Geometry: final body of the model. Coordinates: model frame, mm. A direction names the side the tool comes from. Give positions to 0.01 mm unless a question says otherwise; leave off trailing zeros. Order: outer loops, then holes, each group sorted by start corner. A loop starts at its lowest first (then second) coordinate and runs counter-clockwise, first axis right, second up. Notation, with made-up numbers: (-6.5, 8) - (39.5, 8) arc R28 cw to (39.5, 31) - close; hole circle Ø6 at (23, 81.5). An arc over 180 degrees is marked (long way). Use one line per item in the form item = value.
from build123d import *

# Parameters (mm, degrees)
BOSS_EXTRUDE1_DEPTH = 12.3
SKETCH2_W           = 2.17
SKETCH2_H           = 2.05
CUT_EXTRUDE1_DEPTH  = 4
FILLET1_R           = 2.15
SKETCH4_W           = 3
SKETCH4_H           = 1
BOSS_EXTRUDE2_DEPTH = 1
BOSS_EXTRUDE3_DEPTH = 3
CUT_EXTRUDE2_DEPTH  = 14.994303425


with BuildPart() as part:
    # Sketch1 → Boss-Extrude1 (new body)
    with BuildSketch(Plane(origin=(0, 0, 0), x_dir=(0, 0, -1), z_dir=(1, 0, 0))):
        with BuildLine():
            Line((0, 0.2), (0, 0.4))
            Line((0, 0.4), (0.303108891, 0.575))
            Line((0.303108891, 0.575), (0.303108891, 5.8))
            Line((0.303108891, 5.8), (3.303108891, 5.8))
            Line((3.303108891, 5.8), (3.303108891, 0))
            Line((3.303108891, 0), (0.2, 0))
            ThreePointArc((0.2, 0), (0.058578644, 0.058578644), (0, 0.2))
        make_face()
    extrude(amount=BOSS_EXTRUDE1_DEPTH)

    # Sketch2 → Cut-Extrude1 (cut)
    with BuildSketch(Plane(origin=(0, 5.8, 0), x_dir=(1, 0, 0), z_dir=(0, 1, 0))):
        with Locations((1.085, 2.278108891)):
            Rectangle(SKETCH2_W, SKETCH2_H)
        with Locations((11.215, 2.278108891)):
            Rectangle(SKETCH2_W, SKETCH2_H)
    extrude(amount=-CUT_EXTRUDE1_DEPTH, mode=Mode.SUBTRACT)

    # Fillet1
    fillet1_edges = [part.edges().sort_by_distance(p)[0] for p in [
        (0, 5.8, -0.778108891),
        (12.3, 5.8, -0.778108891),
    ]]
    fillet(fillet1_edges, radius=FILLET1_R)

    # Sketch4 → Boss-Extrude2 (add)
    with BuildSketch(Plane.XY.offset(-0.303108891)):
        with Locations((6.15, 2.55)):
            Rectangle(SKETCH4_W, SKETCH4_H)
    extrude(amount=BOSS_EXTRUDE2_DEPTH)

    # Sketch5 → Boss-Extrude3 (add)
    with BuildSketch(Plane(origin=(7.65, 0, 0), x_dir=(0, 0, -1), z_dir=(1, 0, 0))):
        Polygon((-0.696891109, 3.05), (0.303108891, 3.05), (0.303108891, 4.64), align=None)
    extrude(amount=-BOSS_EXTRUDE3_DEPTH)

    # Sketch7 → Cut-Extrude2 (cut, through all)
    with BuildSketch(Plane(origin=(12.3, 0, 0), x_dir=(0, 0, -1), z_dir=(1, 0, 0))):
        Polygon((3.303108891, 5.8), (3.303108891, 0), (2.683108891, 0), (3.153108891, 5.8), align=None)
    extrude(amount=-CUT_EXTRUDE2_DEPTH, mode=Mode.SUBTRACT)


solid = part.part
(1) Cut plane D-D on x = 4. Output: boundary loops of the cut face in (y, z) (3 decimals), plus the area to 3 significant figures.
Computed values:
outline = (0, -2.683) - (5.8, -3.153) - (5.8, -0.303) - (0.575, -0.303) - (0.4, 0) - (0.2, 0) arc R0.2 ccw to (0, -0.2) - close
area = 15.3 mm²
(2) Cut plane A-A on x = 6.75. Output: boundary loops of the cut face in (y, z) (3 decimals), plus the area to 3 significant figures.
Computed values:
outline = (0, -2.683) - (5.8, -3.153) - (5.8, -0.303) - (4.64, -0.303) - (3.05, 0.697) - (2.05, 0.697) - (2.05, -0.303) - (0.575, -0.303) - (0.4, 0) - (0.2, 0) arc R0.2 ccw to (0, -0.2) - close
area = 17.1 mm²
(3) Cut plane B-B on z = -1.1. Output: boundary loops of the cut face in (x, y), plus the area to 3 significant figures.
Computed values:
outline = (0, 0) - (12.3, 0) - (12.3, 3.65) arc R2.15 ccw to (10.15, 5.8) - (2.15, 5.8) arc R2.15 ccw to (0, 3.65) - close
area = 69.4 mm²
(4) Ray query, line 1 along Y through (x, z) = (11, -1.85); line 2 along X through (y, z) = (3.4, -2.7); line 3 along Z through (x, y) = (11.25, 4.4). Return the intervals inside material, ascending.
Computed values:
line_1 = 0 to 1.8
line_2 = 2.17 to 10.13
line_3 = -1.25 to -0.3
(5) Contact query for flat-ended pins moving along their axis: pin 1 Ø0.5 at (y, z) = (3.5, 0) entering from +X; pin 2 Ø1.5 at (x, y) = (9, 1) entering from -Z; pin 3 Ø0.6 at (y, z) = (4.5, -2.5) entering from +X. Output: stop coordinate, or through.
Computed values:
pin_1 = 7.65
pin_2 = -2.82
pin_3 = 10.13
(6) Cut plane C-C on y = 2.4. Output: boundary loops of the cut face in (x, z), plus the area to 3 significant figures.
Computed values:
outline = (0, -1.25) - (2.17, -1.25) - (2.17, -2.88) - (10.13, -2.88) - (10.13, -1.25) - (12.3, -1.25) - (12.3, -0.3) - (7.65, -0.3) - (7.65, 0.7) - (4.65, 0.7) - (4.65, -0.3) - (0, -0.3) - close
area = 27.6 mm²
(7) Reachability of faces 1 (the face through (4.65, 3, 0)), 2 (the face through (2.17, 4, -2)), 3 (the face through (6, 2.05, 0)) from +Z, -Z, +X, -X, +Y, -Y: full face, straight path, thin tool, end or side. Return the list, or none.
Computed values:
face_1 = +Z, -X, +Y
face_2 = -Z, -X, +Y
face_3 = +Z, +X, -X
